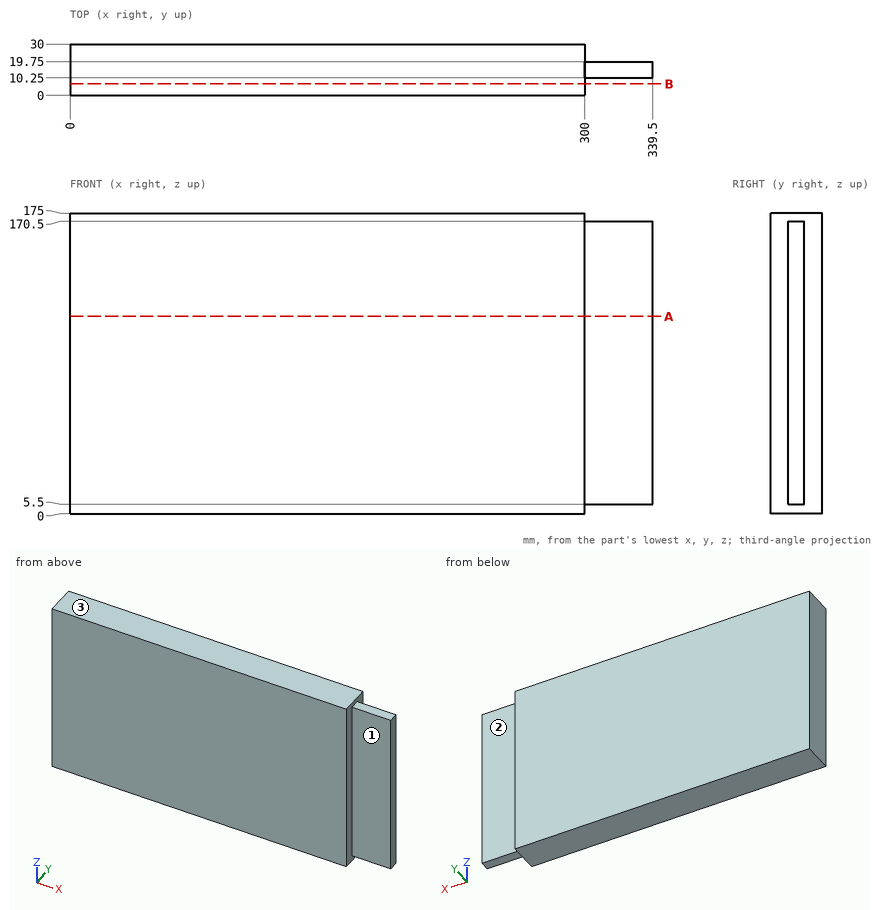
Input: dimensioned drawing with shaded views. Units: mm. Origin: part minimum x, y, z. A direction names the side the tool comes from. Give positions to 0.01 mm unless a question says otherwise; leave off trailing zeros. Write each loop counter-clockwise with the first axis right and the second up, starting at its lowest first coordinate (ties: lowest second). Pieces come first, ordered by that corner, then holes. Notation, with made-up numbers: M 51.25,33 L 89.25,33 A20 cw 89.25,44 Z; hole C 70,-39 d7. An arc over 180 degrees is marked long. Write item = value, one per line. Start each with the question number.
1) First-contact query: pin 1 Ø3 at (x, y) = (327, 15) entering from -Z; pin 2 Ø12 at (x, z) = (310.5, 74.5) entering from -Y; pin 3 Ø5 at (x, y) = (329.5, 13.5) entering from +Z. Flat tips, straight axial feed; report the tip coordinate or a pass-through.
2) Reachability of the marked faces 1, 2 and 3 from +Z, -Z, +X, -X, +Y, -Y: full face, straight path, thin tool, end or side. Return the list, or none.
3) Material intervals for line 1 along X through (y, z) = (5.25, 140), sorted ascending. Write a range as [from, to].
4) Cut plane A-A on z = 115. Return the cut outline in (x, y).
5) Cut plane B-B on y = 6.75. Return the cut outline in (x, z), then the cut area to 3 significant figures.
Solved:
q1.pin_1 = 5.5
q1.pin_2 = 10.25
q1.pin_3 = 170.5
q2.face_1 = +Z, -Z, +X, -Y
q2.face_2 = +Z, -Z, +X, +Y
q2.face_3 = +Z, +X, -X, +Y, -Y
q3.line_1 = [0, 300]
q4.outline = M 0,0 L 300,0 L 300,10.25 L 339.5,10.25 L 339.5,19.75 L 300,19.75 L 300,30 L 0,30 Z
q5.outline = M 0,0 L 300,0 L 300,175 L 0,175 Z
q5.area = 52,500 mm2
